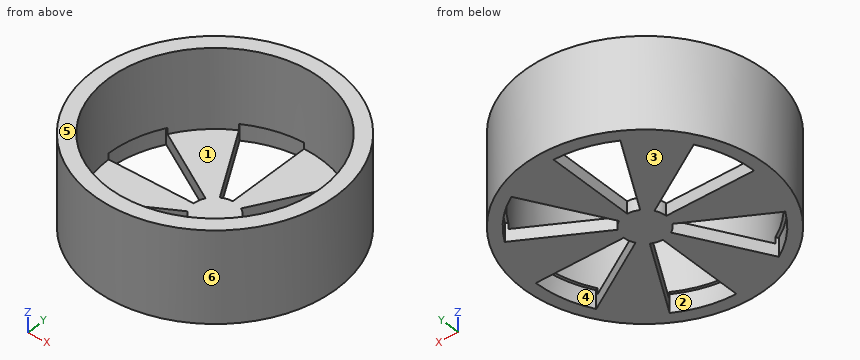
```python
from build123d import *

# Parameters (mm, degrees)
F0_R     = 20
F1_DEPTH = 15
F2_R     = 17.5460358756
F4_DEPTH = 13
F6_DEPTH = 3


# Not quite as in the source:
# - a feature of the source that left no trace in its solid (it failed there, or was rolled back) is left out


with BuildPart() as f1:
    # F0 (on Top) → F1 (new body)
    with BuildSketch(Plane.XY):
        Circle(F0_R)
    extrude(amount=F1_DEPTH)

    # F2 (on face) → F4 (cut)
    with BuildSketch(Plane.XY.offset(15)):
        Circle(F2_R)
    extrude(amount=-F4_DEPTH, mode=Mode.SUBTRACT)

    # F5 (on face) → F6 (cut)
    with BuildSketch(Plane.XY):
        with BuildLine():
            ThreePointArc((0, -18), (4.6587428118, -17.3866648732), (9, -15.5884572681))
            Line((9, -15.5884572681), (1.75, -3.0310889132))
            ThreePointArc((1.75, -3.0310889132), (0.9058666579, -3.380740392), (0, -3.5))
            Line((0, -3.5), (0, -18))
        make_face()
        with BuildLine():
            ThreePointArc((15.5884572681, -9), (17.3866648732, -4.6587428118), (18, 0))
            Line((18, 0), (3.5, 0))
            ThreePointArc((3.5, 0), (3.380740392, -0.9058666579), (3.0310889132, -1.75))
            Line((3.0310889132, -1.75), (15.5884572681, -9))
        make_face()
        with BuildLine():
            Line((3.0310889132, 1.75), (15.5884572681, 9))
            ThreePointArc((15.5884572681, 9), (12.7279220614, 12.7279220614), (9, 15.5884572681))
            Line((9, 15.5884572681), (1.75, 3.0310889132))
            ThreePointArc((1.75, 3.0310889132), (2.4748737342, 2.4748737342), (3.0310889132, 1.75))
        make_face()
        with BuildLine():
            Line((0, 3.5), (0, 18))
            ThreePointArc((0, 18), (-4.6587428118, 17.3866648732), (-9, 15.5884572681))
            Line((-9, 15.5884572681), (-1.75, 3.0310889132))
            ThreePointArc((-1.75, 3.0310889132), (-0.9058666579, 3.380740392), (0, 3.5))
        make_face()
        with BuildLine():
            Line((-3.0310889132, 1.75), (-15.5884572681, 9))
            ThreePointArc((-15.5884572681, 9), (-17.3866648732, 4.6587428118), (-18, 0))
            Line((-18, 0), (-3.5, 0))
            ThreePointArc((-3.5, 0), (-3.380740392, 0.9058666579), (-3.0310889132, 1.75))
        make_face()
        with BuildLine():
            ThreePointArc((-15.5884572681, -9), (-12.7279220614, -12.7279220614), (-9, -15.5884572681))
            Line((-9, -15.5884572681), (-1.75, -3.0310889132))
            ThreePointArc((-1.75, -3.0310889132), (-2.4748737342, -2.4748737342), (-3.0310889132, -1.75))
            Line((-3.0310889132, -1.75), (-15.5884572681, -9))
        make_face()
    extrude(amount=F6_DEPTH, mode=Mode.SUBTRACT)


solid = f1.part
```
Here's how the part is built. I have some questions about the finished solid (model axes, mm). Face numbers are marked on the shaded views. A direction names the side the tool comes from. Give positions to 0.01 mm unless a question says otherwise; leave off trailing zeros. Order: outer loops, then holes, each group sorted by start corner. A loop starts at its lowest first (then second) coordinate and runs counter-clockwise, first axis right, second up. Notation, with made-up numbers: (-12, 85.5) -> (7, 85.5) arc R19 cw to (7, 97.5) -> close; hole circle Ø8 at (-29.5, 45.25). An arc over 180 degrees is marked (long way). Use CSV: the item, a comma, the result in double quotes. Start each with the question number.
Item 1: Suppose I cut it at C-C (y = 13.5). List the corners of the cut face in (x, z) for me, and give its area (3 significant figures).
Item 2: Suppose I cut it at B-B (x = -4). List the corners of the cut face in (y, z) for me, and give its area (3 significant figures).
Item 3: I'm going to push flat-ended pins straight in: P1, Ø6, axis at y = -12.5, z = 9, coming from the +X side; P2, Ø2.5, axis at y = 12, z = 1.5, coming from the -X side; P3, Ø4, axis at y = -12, z = 13, coming from the +X side. Where does each tip first touch, or does it pass through?
Item 4: If I drill on probe 1 along Y at (x, z) = (0, 11.75); probe 2 along X at (y, z) = (-1, 2.5); probe 3 along X at (y, z) = (-16, 9), over which ranges is the centre line in solid material (lowest first)? Write a range as [from, to].
Item 5: Thinking about a two-plate mould opening in Y: for the marked faces 4, 5 and 6, which applies, pulls with the +Y half, pulls with the -Y half, needs draft (parallel to the pull), parting line crosses it, or undercut?
Item 6: Suppose I cut it at A-A (y = 5.5). List the corners of the cut face in (x, z) for me, and give its area (3 significant figures).
Item 7: Suppose I cut it at D-D (z = 9.5). List the corners of the cut face in (x, y) for me, and give its area (3 significant figures).
Item 8: On a 3-axis mill with a long thin cutter (end or side, diameter ignored), from which of +Z, -Z, +X, -X, +Y, -Y can I reach the whole of each face in a straight line? I mean the marked faces 1, 2 and 3. Say none if no direction works.
Answer block:
1,outline,"(-14.76, 0) -> (-7.79, 0) -> (-7.79, 2) -> (-11.21, 2) -> (-11.21, 15) -> (-14.76, 15) -> close; (0, 0) -> (7.79, 0) -> (7.79, 2) -> (0, 2) -> close; (11.21, 3) -> (11.91, 3) -> (11.91, 0) -> (14.76, 0) -> (14.76, 15) -> (11.21, 15) -> close"
1,area,"127 mm^2"
2,outline,"(-19.6, 0) -> (-6.93, 0) -> (-6.93, 2) -> (-17.08, 2) -> (-17.08, 15) -> (-19.6, 15) -> close; (-2.31, 0) -> (0, 0) -> (0, 2) -> (-2.31, 2) -> close; (2.31, 0) -> (6.93, 0) -> (6.93, 2) -> (2.31, 2) -> close; (17.08, 3) -> (17.55, 3) -> (17.55, 0) -> (19.6, 0) -> (19.6, 15) -> (17.08, 15) -> close"
2,area,"108 mm^2"
3,P1,"stops at x = 17.6"
3,P2,"stops at x = -16.87"
3,P3,"stops at x = 17.32"
4,probe 1,"y = [-20, -17.55], [17.55, 20]"
4,probe 2,"x = [-19.97, -17.52], [17.97, 19.97]"
4,probe 3,"x = [-12, -7.2], [7.2, 12]"
5,face 4,"undercut"
5,face 5,"needs draft"
5,face 6,"parting line crosses it"
6,outline,"(-19.23, 0) -> (-17.14, 0) -> (-17.14, 3) -> (-16.66, 3) -> (-16.66, 15) -> (-19.23, 15) -> close; (-9.53, 0) -> (-3.18, 0) -> (-3.18, 2) -> (-9.53, 2) -> close; (0, 0) -> (3.18, 0) -> (3.18, 2) -> (0, 2) -> close; (9.53, 0) -> (19.23, 0) -> (19.23, 15) -> (16.66, 15) -> (16.66, 2) -> (9.53, 2) -> close"
6,area,"109 mm^2"
7,outline,"circle Ø40 at (0, 0); hole circle Ø35.09 at (0, 0)"
7,area,"289 mm^2"
8,face 1,"+Z"
8,face 2,"-Z"
8,face 3,"-Z, +X, -X, +Y, -Y"
